Input: part model. Units: mm. Frame: model coordinates. A direction names the side the tool comes from. Round coordinates to 2 decimals unless told otherwise and drop trailing zeros. Loops run counter-clockwise (first coordinate to the right, second up) from the corner with the lowest first, then second, coordinate; pieces in that order, holes last. Notation, with made-up numbers: (5.25, 55.25) -> (41.25, 55.25) arc R9 ccw to (41.25, 69.25) -> close; hole circle Ø8 at (21.5, -26.5). An arc over 180 degrees is marked (long way). Answer as a JSON object with one key per item and string values.
```python
from build123d import *

# Parameters (mm, degrees)
F0_W     = 1380
F0_H     = 700
F0_W_2   = 1180
F0_H_2   = 500
F1_DEPTH = 100
F2_W     = 1180
F2_H     = 500
F3_DEPTH = 300
F4_R     = 55
F5_DEPTH = 1819
F6_DEPTH = 400.001
F8_DEPTH = 100


# Not quite as in the source:
# - an extrude ends at something that could not be found from the text; its depth is read off the source's solid
# - a feature of the source that left no trace in its solid (it failed there, or was rolled back) is left out


with BuildPart() as f1:
    # F0 (on Top) → F1 (new body)
    with BuildSketch(Plane.XY):
        Rectangle(F0_W, F0_H)
        Rectangle(F0_W_2, F0_H_2, mode=Mode.SUBTRACT)
        Rectangle(F0_W_2, F0_H_2)
    extrude(amount=F1_DEPTH)

    # F2 (on face) → F3 (join)
    with BuildSketch(Plane.XY.offset(100)):
        with Locations((1.1069327593, 0)):
            Rectangle(F2_W, F2_H)
    extrude(amount=F3_DEPTH)

    # F4 (on face) → F5 (cut, through all)
    with BuildSketch(Plane.XY.offset(400)):
        with BuildLine():
            ThreePointArc((-340, 150), (-490, 0), (-340, -150))
            Line((-340, -150), (340, -150))
            ThreePointArc((340, -150), (490, 0), (340, 150))
            Line((340, 150), (-340, 150))
        make_face()
        with Locations((-340, 0)):
            Circle(F4_R, mode=Mode.SUBTRACT)
        with Locations((340, 0)):
            Circle(F4_R, mode=Mode.SUBTRACT)
    extrude(amount=F5_DEPTH, mode=Mode.SUBTRACT)

    # F4 (on face) → F6 (cut, through all)
    with BuildSketch(Plane.XY.offset(400)):
        with BuildLine():
            ThreePointArc((-340, 150), (-490, 0), (-340, -150))
            Line((-340, -150), (340, -150))
            ThreePointArc((340, -150), (490, 0), (340, 150))
            Line((340, 150), (-340, 150))
        make_face()
        with Locations((-340, 0)):
            Circle(F4_R, mode=Mode.SUBTRACT)
        with Locations((340, 0)):
            Circle(F4_R, mode=Mode.SUBTRACT)
    extrude(amount=-F6_DEPTH, mode=Mode.SUBTRACT)

    # F4 (on face) → F8 (join)
    with BuildSketch(Plane.XY.offset(400)):
        with BuildLine():
            ThreePointArc((-340, 150), (-490, 0), (-340, -150))
            Line((-340, -150), (340, -150))
            ThreePointArc((340, -150), (490, 0), (340, 150))
            Line((340, 150), (-340, 150))
        make_face()
        with Locations((-340, 0)):
            Circle(F4_R, mode=Mode.SUBTRACT)
        with Locations((340, 0)):
            Circle(F4_R, mode=Mode.SUBTRACT)
        with Locations((-340, 0)):
            Circle(F4_R)
        with Locations((340, 0)):
            Circle(F4_R)
    extrude(amount=-F8_DEPTH)


solid = f1.part
```
1) Section D-D, the plane z = 368.5. Output: boundary loops of the cut face in (x, y), plus the area to 3 significant figures.
Output:
{"outline": "(-588.89, -250) -> (591.11, -250) -> (591.11, 250) -> (-588.89, 250) -> close", "area": "590,000 mm^2"}
2) Draft query along X for faces 6 (the face through (-5, -150, 152)), 7 (the face through (-10, 160, 0)), 8 (the face through (-690, -5, 49)), 9 (the face through (-289.194, -21.065, 152.1)). Return one class per face: +X half, -X half, draft (parallel to the pull), parting line (faces both ways), or undercut.
Output:
{"face 6": "undercut", "face 7": "draft", "face 8": "-X half", "face 9": "undercut"}
3) Section A-A, the plane z = 171.5. Output: boundary loops of the cut face in (x, y), plus the area to 3 significant figures.
Output:
{"outline": "(-588.89, -250) -> (591.11, -250) -> (591.11, 250) -> (-588.89, 250) -> close; circle Ø110 at (-340, 0); circle Ø110 at (340, 0); hole (-340, -150) -> (340, -150) arc R150 ccw to (340, 150) -> (-340, 150) arc R150 ccw to start", "area": "334,000 mm^2"}
4) Section B-B, the plane x = 539.5. Output: boundary loops of the cut face in (y, z).
Output:
{"outline": "(-350, 0) -> (350, 0) -> (350, 100) -> (250, 100) -> (250, 400) -> (-250, 400) -> (-250, 100) -> (-350, 100) -> close"}
5) Section C-C, the plane y = -216.5. Output: boundary loops of the cut face in (x, z).
Output:
{"outline": "(-690, 0) -> (690, 0) -> (690, 100) -> (591.11, 100) -> (591.11, 400) -> (-588.89, 400) -> (-588.89, 100) -> (-690, 100) -> close"}
6) Contact query for flat-ended pins moving along their axis: P1, Ø4, axis at x = -166, z = 149.5, coming from the -Y side; P2, Ø3, axis at y = 142, z = 121.5, coming from the -X side; P3, Ø6, axis at x = -169, y = 277.5, coming from the +Z side. Output: stop coordinate, or through.
Output:
{"P1": "stops at y = -250", "P2": "stops at x = -588.89", "P3": "stops at z = 100"}
7) Ray query, probe 1 along Y at (x, z) = (-329, 212.5); probe 2 along Y at (x, z) = (296, 205.5); probe 3 along Y at (x, z) = (208, 195). Return the intervals inside material, ascending.
Output:
{"probe 1": "y = -250 to -150, -53.89 to 53.89, 150 to 250", "probe 2": "y = -250 to -150, -33 to 33, 150 to 250", "probe 3": "y = -250 to -150, 150 to 250"}
8) Reachability of faces 1 (the face through (591.107, -3, 248)), 2 (the face through (-588.893, -3, 248)), 3 (the face through (-7, -250, 248)), 4 (the face through (-7, 250, 248)), 5 (the face through (-7, 2, 300)) from +Z, -Z, +X, -X, +Y, -Y: full face, straight path, thin tool, end or side. Return the list, or none.
Output:
{"face 1": "+Z, +X, +Y, -Y", "face 2": "+Z, -X, +Y, -Y", "face 3": "+Z, +X, -X, -Y", "face 4": "+Z, +X, -X, +Y", "face 5": "-Z"}
